Build history of the part. All positions in model axes, mm. A direction names the side the tool comes from. Coordinates: 2 decimals unless noted, no trailing zeros. One line per item, written item: value.
```python
from build123d import *

# Parameters (mm, degrees)
PLACA_INFERIOR_1_2IN_DEPTH              = 12.7
CROQUIS20_R                             = 2.75
ANCLAJES_4XM5_DEPTH                     = 12.7
CROQUIS21_R                             = 1.7
CROQUIS21_R_2                           = 1.45
BARRENOS_M3_PAREDES_Y_M2_5_POSTES_DEPTH = 12.7
CROQUIS22_R                             = 2.9
REFRENTADO_M3_INFERIOR_DEPTH            = 3.2
CROQUIS23_R                             = 2.5
REFRENTADO_M2_5_INFERIOR_DEPTH          = 2.6


with BuildPart() as part:
    # Croquis19 → Placa_inferior_1-2in (new body)
    with BuildSketch(Plane.XY):
        with BuildLine():
            Line((-144.7, -116.6), (93.9, -116.6))
            ThreePointArc((93.9, -116.6), (100.971067812, -113.671067812), (103.9, -106.6))
            Line((103.9, -106.6), (103.9, 106.6))
            ThreePointArc((103.9, 106.6), (100.971067812, 113.671067812), (93.9, 116.6))
            Line((93.9, 116.6), (-144.7, 116.6))
            ThreePointArc((-144.7, 116.6), (-151.771067812, 113.671067812), (-154.7, 106.6))
            Line((-154.7, 106.6), (-154.7, -106.6))
            ThreePointArc((-154.7, -106.6), (-151.771067812, -113.671067812), (-144.7, -116.6))
        make_face()
    extrude(amount=PLACA_INFERIOR_1_2IN_DEPTH)

    # Croquis20 → Anclajes_4xM5 (cut)
    with BuildSketch(Plane.XY):
        with Locations((-147.2, -109.1)):
            Circle(CROQUIS20_R)
        with Locations((-147.2, 109.1)):
            Circle(CROQUIS20_R)
        with Locations((96.4, -109.1)):
            Circle(CROQUIS20_R)
        with Locations((96.4, 109.1)):
            Circle(CROQUIS20_R)
    extrude(amount=ANCLAJES_4XM5_DEPTH, mode=Mode.SUBTRACT)

    # Croquis21 → Barrenos_M3_paredes_y_M2-5_postes (cut)
    with BuildSketch(Plane.XY):
        with Locations((-125, 98.425)):
            Circle(CROQUIS21_R)
        with Locations((-125, -98.425)):
            Circle(CROQUIS21_R)
        with Locations((-30, 98.425)):
            Circle(CROQUIS21_R)
        with Locations((-30, -98.425)):
            Circle(CROQUIS21_R)
        with Locations((70, 98.425)):
            Circle(CROQUIS21_R)
        with Locations((70, -98.425)):
            Circle(CROQUIS21_R)
        with Locations((-136.525, -50)):
            Circle(CROQUIS21_R)
        with Locations((-136.525, 50)):
            Circle(CROQUIS21_R)
        with Locations((85.725, -50)):
            Circle(CROQUIS21_R)
        with Locations((85.725, 50)):
            Circle(CROQUIS21_R)
        with Locations((-108.5, -56)):
            Circle(CROQUIS21_R_2)
        with Locations((-108.5, 2)):
            Circle(CROQUIS21_R_2)
        with Locations((-59.5, -56)):
            Circle(CROQUIS21_R_2)
        with Locations((-59.5, 2)):
            Circle(CROQUIS21_R_2)
    extrude(amount=BARRENOS_M3_PAREDES_Y_M2_5_POSTES_DEPTH, mode=Mode.SUBTRACT)

    # Croquis22 → Refrentado_M3_inferior (cut)
    with BuildSketch(Plane.XY):
        with Locations((-125, 98.425)):
            Circle(CROQUIS22_R)
        with Locations((-125, -98.425)):
            Circle(CROQUIS22_R)
        with Locations((-30, 98.425)):
            Circle(CROQUIS22_R)
        with Locations((-30, -98.425)):
            Circle(CROQUIS22_R)
        with Locations((70, 98.425)):
            Circle(CROQUIS22_R)
        with Locations((70, -98.425)):
            Circle(CROQUIS22_R)
        with Locations((-136.525, -50)):
            Circle(CROQUIS22_R)
        with Locations((-136.525, 50)):
            Circle(CROQUIS22_R)
        with Locations((85.725, -50)):
            Circle(CROQUIS22_R)
        with Locations((85.725, 50)):
            Circle(CROQUIS22_R)
    extrude(amount=REFRENTADO_M3_INFERIOR_DEPTH, mode=Mode.SUBTRACT)

    # Croquis23 → Refrentado_M2-5_inferior (cut)
    with BuildSketch(Plane.XY):
        with Locations((-108.5, -56)):
            Circle(CROQUIS23_R)
        with Locations((-108.5, 2)):
            Circle(CROQUIS23_R)
        with Locations((-59.5, -56)):
            Circle(CROQUIS23_R)
        with Locations((-59.5, 2)):
            Circle(CROQUIS23_R)
    extrude(amount=REFRENTADO_M2_5_INFERIOR_DEPTH, mode=Mode.SUBTRACT)


solid = part.part
```
Item 1: Drop flat-ended pins along their axis: P1, Ø2.5, axis at x = -59, y = -55, coming from the -Z side; P2, Ø1.7, axis at x = -126, y = 99, coming from the -Z side. Give the stop position or say it passes through.
Check result:
P1: stops at z = 2.6
P2: stops at z = 3.2
Item 2: Pull direction X, two halves, no side cores. Call faces 3 (the face through (101.05, 113.59, 6.26)), 4 (the face through (-154.7, 1, 6)), 5 (the face through (99.02, -108.27, 6.26)): released by +X, released by -X, zero draft, split by the parting line, or undercut.
Check result:
face 3: released by +X
face 4: released by -X
face 5: undercut
Item 3: Tool access for faces 1 (the face through (-127.3, -100.19, 1.58)), 2 (the face through (-151.69, 113.75, 6.26)): list every direction of +Z, -Z, +X, -X, +Y, -Y with a clear straight run to the whole face (end or side of a thin tool).
Check result:
face 1: -Z
face 2: +Z, -Z, -X, +Y
Item 4: Probe probe 1 along Y at (x, z) = (-125, 8.5) (3 decimals); probe 2 along Y at (x, z) = (-137, 3.25); probe 3 along X at (y, z) = (1, 10.5). List the from-to ranges inside material, lowest first. Write a range as from..to.
Check result:
probe 1: y = -116.6..-100.125, -96.725..96.725, 100.125..116.6
probe 2: y = -116.6..-51.63, -48.37..48.37, 51.63..116.6
probe 3: x = -154.7..-109.55, -107.45..-60.55, -58.45..103.9
